Verification items for the finished model (mm, model axes). A direction names the side the tool comes from. Round coordinates to 2 decimals unless told otherwise and drop trailing zeros. Write each loop counter-clockwise with the first axis right and the second up, starting at its lowest first coordinate (ties: lowest second). Pieces come first, ordered by that corner, then holes. Notation, with made-up numbers: (4.5, 56) - (59.5, 56) arc R7 ccw to (59.5, 69) - close; hole circle Ø1 at (39, 16). An arc over 180 degrees is marked (long way). Write each question's results on one line, items separated by ' | '.
```python
from build123d import *

# Parameters (mm, degrees)
SKETCH1_W           = 40
SKETCH1_H           = 90
BOSS_EXTRUDE1_DEPTH = 5
SKETCH2_W           = 40
SKETCH2_H           = 20
BOSS_EXTRUDE2_DEPTH = 30
SKETCH3_R           = 10
CUT_EXTRUDE1_DEPTH  = 30


with BuildPart() as part:
    # Sketch1 → Boss-Extrude1 (new body)
    with BuildSketch(Plane.XY):
        with Locations((-0.107274634, 14.603113743)):
            Rectangle(SKETCH1_W, SKETCH1_H)
    extrude(amount=BOSS_EXTRUDE1_DEPTH)

    # Sketch2 → Boss-Extrude2 (add)
    with BuildSketch(Plane.XY.offset(5)):
        with Locations((-0.107274634, -20.396886257)):
            Rectangle(SKETCH2_W, SKETCH2_H)
    extrude(amount=BOSS_EXTRUDE2_DEPTH)

    # Sketch3 → Cut-Extrude1 (cut)
    with BuildSketch(Plane(origin=(0, 0, 0), x_dir=(-1, 0, 0), z_dir=(0, 0, -1))):
        with Locations((0.107274634, 34.603113743)):
            Circle(SKETCH3_R)
    extrude(amount=-CUT_EXTRUDE1_DEPTH, mode=Mode.SUBTRACT)


solid = part.part
```
(1) Thickness scan on L1, parallel to Y at x = 10.5, z = 16; L2, parallel to Z at x = -2, y = 11. Record the ranges inside material, lowest first.
Answer:
L1: -30.4 to -10.4 | L2: 0 to 5
(2) Section check A-A (x = 1). Record the cut outline in (y, z), plus the area to 3 significant figures.
Answer:
outline: (-30.4, 0) - (24.66, 0) - (24.66, 5) - (-10.4, 5) - (-10.4, 35) - (-30.4, 35) - close; (44.54, 0) - (59.6, 0) - (59.6, 5) - (44.54, 5) - close | area: 951 mm2
(3) Section check D-D (y = 12). Record the cut outline in (x, z), plus the area to 3 significant figures.
Answer:
outline: (-20.11, 0) - (19.89, 0) - (19.89, 5) - (-20.11, 5) - close | area: 200 mm2
(4) Set-up check for faces 1 (the flat face through (0, -20, 35)), 2 (the flat face through (-5, 25, 5)): record each of +Z, -Z, +X, -X, +Y, -Y from which the full face is reachable in a straight line by a thin tool's end or side.
Answer:
face 1: +Z, +X, -X, +Y, -Y | face 2: +Z, +X, -X, +Y
(5) Mould release check, pull along X, two halves, no side actions. Record for faces 3 (the cylindrical face through (2.06, 24.84, 2.46)), 4 (the flat face through (-20.107, -12, 14)), 5 (the flat face through (0, -10.397, 20)), 6 (the flat face through (19.893, -12, 14)): released by +X, released by -X, zero draft, split by the parting line, or undercut.
Answer:
face 3: undercut | face 4: released by -X | face 5: zero draft | face 6: released by +X
(6) Go/stop test with flat-tipped pins: pin 1 Ø6 at (x, y) = (6.5, 25) entering from +Z; pin 2 Ø12 at (x, y) = (1.5, 33) entering from +Z; pin 3 Ø4 at (x, z) = (4.5, 22.5) entering from +Y; pin 4 Ø2 at (x, y) = (-3.5, -13) entering from -Z. Record where each tip stops, or that it passes through.
Answer:
pin 1: z = 5 | pin 2: through | pin 3: y = -10.4 | pin 4: z = 0
(7) Section check B-B (x = -14). Record the cut outline in (y, z).
Answer:
outline: (-30.4, 0) - (59.6, 0) - (59.6, 5) - (-10.4, 5) - (-10.4, 35) - (-30.4, 35) - close
(8) Section check C-C (z = 28). Record the cut outline in (x, y).
Answer:
outline: (-20.11, -30.4) - (19.89, -30.4) - (19.89, -10.4) - (-20.11, -10.4) - close
